from build123d import *

# Parameters (mm, degrees)
BOSS_EXTRUDE1_DEPTH = 10
FILLET1_R           = 1
SKETCH2_W           = 21.86553483
SKETCH2_H           = 30.5
CUT_EXTRUDE1_DEPTH  = 5
MIRROR1_DEPTH       = 10
MIRROR1_2_OUTLINE_W = 21.86553483
MIRROR1_2_OUTLINE_H = 30.5
MIRROR1_2_DEPTH     = 5
SKETCH6_W           = 35.925
SKETCH6_H           = 8.5
CUT_EXTRUDE2_DEPTH  = 10


# Read off the part's stored shape, not the designer's step: Mirror1
with BuildPart() as part:
    # Sketch1 → Boss-Extrude1 (new body)
    with BuildSketch(Plane(origin=(0, 0, 0), x_dir=(1, 0, 0), z_dir=(0, 1, 0))):
        Polygon((-5, 57.097150921), (34.3, 57.097150921), (34.3, 55.097150921), (31.675, 55.097150921), (31.675, 52.597150921), (31.675, 2.599340873), (31.675, 0.099340873), (34.3, 0.099340873), (34.3, -4.5), (-5, -4.5), align=None)
        Polygon((-2.625, 45), (-2.625, 0), (-2.625, -2.5), (0, -2.5), (2.625, -2.5), (2.625, 0), (2.625, 45), (2.625, 47.5), (0, 47.5), (-2.625, 47.5), align=None, mode=Mode.SUBTRACT)
    extrude(amount=BOSS_EXTRUDE1_DEPTH)

    # Fillet1
    fillet1_edges = [part.edges().sort_by_distance(p)[0] for p in [
        (31.675, 5, -55.097150921),
        (31.675, 5, -0.099340873),
        (-2.625, 5, -47.5),
        (-2.625, 5, 2.5),
        (2.625, 5, 2.5),
        (2.625, 5, -47.5),
    ]]
    fillet(fillet1_edges, radius=FILLET1_R)

    # Sketch2 → Cut-Extrude1 (cut)
    with BuildSketch(Plane(origin=(0, 10, 0), x_dir=(1, 0, 0), z_dir=(0, 1, 0))):
        with Locations((20.742232585, 23.8519351)):
            Rectangle(SKETCH2_W, SKETCH2_H)
    extrude(amount=-CUT_EXTRUDE1_DEPTH, mode=Mode.SUBTRACT)

    # Mirror1 outline → Mirror1 (add)
    with BuildSketch(Plane(origin=(0, 0, 0), x_dir=(1, 0, 0), z_dir=(0, 1, 0))):
        with BuildLine():
            ThreePointArc((35.925, 55.097150921), (36.632106781, 54.804257702), (36.925, 54.097150921))
            Line((36.925, 54.097150921), (36.925, 39.1019351))
            Line((36.925, 39.1019351), (58.79053483, 39.1019351))
            Line((58.79053483, 39.1019351), (58.79053483, 8.6019351))
            Line((58.79053483, 8.6019351), (36.925, 8.6019351))
            Line((36.925, 8.6019351), (36.925, 1.099340873))
            ThreePointArc((36.925, 1.099340873), (36.632106781, 0.392234092), (35.925, 0.099340873))
            Line((35.925, 0.099340873), (34.3, 0.099340873))
            Line((34.3, 0.099340873), (34.3, -4.5))
            Line((34.3, -4.5), (73.6, -4.5))
            Line((73.6, -4.5), (73.6, 57.097150921))
            Line((73.6, 57.097150921), (34.3, 57.097150921))
            Line((34.3, 57.097150921), (34.3, 55.097150921))
            Line((34.3, 55.097150921), (35.925, 55.097150921))
        make_face()
        with BuildLine():
            Line((70.225, -2.5), (66.975, -2.5))
            ThreePointArc((66.975, -2.5), (66.267893219, -2.207106781), (65.975, -1.5))
            Line((65.975, -1.5), (65.975, 46.5))
            ThreePointArc((65.975, 46.5), (66.267893219, 47.207106781), (66.975, 47.5))
            Line((66.975, 47.5), (70.225, 47.5))
            ThreePointArc((70.225, 47.5), (70.932106781, 47.207106781), (71.225, 46.5))
            Line((71.225, 46.5), (71.225, -1.5))
            ThreePointArc((71.225, -1.5), (70.932106781, -2.207106781), (70.225, -2.5))
        make_face(mode=Mode.SUBTRACT)
    extrude(amount=MIRROR1_DEPTH)

    # Mirror1 2 outline → Mirror1 2 (add)
    with BuildSketch(Plane(origin=(0, 0, 0), x_dir=(1, 0, 0), z_dir=(0, 1, 0))):
        with Locations((47.857767415, 23.8519351)):
            Rectangle(MIRROR1_2_OUTLINE_W, MIRROR1_2_OUTLINE_H)
    extrude(amount=MIRROR1_2_DEPTH)

    # Sketch6 → Cut-Extrude2 (cut)
    with BuildSketch(Plane(origin=(0, 10, 0), x_dir=(1, 0, 0), z_dir=(0, 1, 0))):
        with Locations((12.9625, -0.25)):
            Rectangle(SKETCH6_W, SKETCH6_H)
        Polygon((73.6, 57.097150921), (66.19379908, 57.097150921), (73.6, 51.534362721), align=None)
    extrude(amount=-CUT_EXTRUDE2_DEPTH, mode=Mode.SUBTRACT)


solid = part.part
Source: CAD feature listing. Evaluate the final solid. Frame: model axes, mm. A direction names the side the tool comes from. Round coordinates to 2 decimals unless told otherwise and drop trailing zeros. Loops run counter-clockwise (first coordinate to the right, second up) from the corner with the lowest first, then second, coordinate; pieces in that order, holes last.
Q1. Mould query, pull axis Z, two halves, no side actions, for faces 1 (the face through (48, 5, -24)), 2 (the face through (42, 10, -40)), 3 (the face through (31, 5, -57.097)). Classes: pulls with the +Z half, pulls with the -Z half, needs draft (parallel to the pull), parting line crosses it, or undercut.
Q2. Ray query, line 1 (X direction, y = 5.5, z = -30.5) (3 decimals); line 2 (X direction, y = 4, z = -32) (3 decimals); line 3 (Z direction, x = 33, y = 7.5). Return the intervals inside material, ascending.
Q3. Section A-A, the plane x = 35. Return loops of the section in (y, z).
Q4. Access query for faces 4 (the face through (34, 5, -0.099)), 5 (the face through (-2.625, 5, -25)), 6 (the face through (21, 8, -8.602)), 7 (the face through (-4, 5, -4)). Directions: +Z, -Z, +X, -X, +Y, -Y. A direction counts if a zero-diameter tool reaches every point of the face in a straight line with its end or side. Return the directions, or none.
Q5. Section C-C, the plane y = 1.75. State how many separate pieces and enclosed holes the cut face has, plus the area to 3 significant figures.
Q6. Section B-B, the plane z = -49. Return loops of the section in (x, y) (3 decimals), plus the area to 4 significant figures.
Q7. First-contact query: P1, Ø24, axis at x = 53, z = -24.5, coming from the +Y side; P2, Ø2.5, axis at x = -3.5, y = 5, coming from the +Z side; P3, Ø1.5, axis at x = 38, z = -37, coming from the +Y side; P4, Ø2.5, axis at x = 68, y = 7, coming from the -Z side. Flat tips, straight axial feed; report the tip coordinate or a pass-through.
Q8. Section D-D, the plane z = -36. Return loops of the section in (x, y) (3 decimals), plus the area to 3 significant figures.
Solutions:
1. face 1: undercut
1. face 2: needs draft
1. face 3: pulls with the -Z half
2. line 1: x = -5 to -2.625, 2.625 to 9.809, 58.791 to 65.975, 71.225 to 73.6
2. line 2: x = -5 to -2.625, 2.625 to 31.675, 36.925 to 65.975, 71.225 to 73.6
2. line 3: z = -57.1 to -55.1, -0.1 to 4.5
3. outline: (0, -57.1) - (10, -57.1) - (10, -55.1) - (0, -55.1) - close; (0, -0.1) - (10, -0.1) - (10, 4.5) - (0, 4.5) - close
4. face 4: +Y, -Y
4. face 5: +Z, +Y, -Y
4. face 6: +Y
4. face 7: +Z, -X, +Y, -Y
5. separate pieces: 1
5. enclosed holes: 2
5. area: 3,740 mm2
6. outline: (-5, 0) - (31.675, 0) - (31.675, 10) - (-5, 10) - close; (36.925, 0) - (73.6, 0) - (73.6, 10) - (36.925, 10) - close
6. area: 733.5 mm2
7. P1: stops at y = 10
7. P2: stops at z = -4
7. P3: stops at y = 5
7. P4: stops at z = -56.68
8. outline: (-5, 0) - (-2.625, 0) - (-2.625, 10) - (-5, 10) - close; (2.625, 0) - (31.675, 0) - (31.675, 5) - (9.809, 5) - (9.809, 10) - (2.625, 10) - close; (36.925, 0) - (65.975, 0) - (65.975, 10) - (58.791, 10) - (58.791, 5) - (36.925, 5) - close; (71.225, 0) - (73.6, 0) - (73.6, 10) - (71.225, 10) - close
8. area: 410 mm2
